The model under review builds one solid part; all positions refer to its coordinate system, in mm. A direction names the side the tool comes from. Round coordinates to 2 decimals unless told otherwise and drop trailing zeros. Write each loop counter-clockwise with the first axis right and the second up, starting at its lowest first coordinate (ties: lowest second). Pieces come first, ordered by that corner, then holes. Notation, with made-up numbers: (73, 59) - (111, 59) arc R18 ccw to (111, 91) - close; hole circle Ø4 at (-32.75, 71.5). An arc over 180 degrees is marked (long way). Use one line per item in the form item = value.
Autodesk Inventor part; units mm, degrees
ref_plane "YZ Plane" through (0, 0, 0) normal (1, 0, 0) x (0, 1, 0)
ref_plane "XZ Plane" through (0, 0, 0) normal (0, 1, 0) x (-1, 0, 0)
ref_plane "XY Plane" through (0, 0, 0) normal (0, 0, 1) x (1, 0, 0)
sketch "Sketch1" plane through (0, 0, 0) normal (0, 1, 0) x (-1, 0, 0)
  line L0 (0, 0) -> (-200, 0)
  line L1 (-200, 0) -> (-200, -150)
  line L2 (-200, -150) -> (0, -150)
  line L3 (0, -150) -> (0, 0)
  line L4 (-109.8726, -150) -> (-90.1274, -150)
  line L5 (-200, -85.1274) -> (-200, -64.8726)
  line L6 (-186.0054, -60.2304) -> (-186.0054, -75)
  line L7 (-200, -64.8726) -> (-187.7125, -59.1428)
  arc A0 (-186.0054, -60.2304) -> (-187.7125, -59.1428) centre (-187.2054, -60.2304) ccw
  line L8 (-186.0054, -75) -> (-186.0054, -89.7696)
  line L9 (-199.8, -85) -> (-186.3697, -85) construction
  arc A1 (-187.7125, -90.8572) -> (-186.0054, -89.7696) centre (-187.2054, -89.7696) ccw
  line L10 (-187.7125, -90.8572) -> (-200, -85.1274)
  line L11 (-89.8726, -150) -> (-110.1274, -150)
  line L12 (-114.7696, -136.0054) -> (-100, -136.0054)
  line L13 (-110.1274, -150) -> (-115.8572, -137.7125)
  arc A2 (-114.7696, -136.0054) -> (-115.8572, -137.7125) centre (-114.7696, -137.2054) ccw
  line L14 (-100, -136.0054) -> (-85.2304, -136.0054)
  line L15 (-90, -149.8) -> (-90, -136.3697) construction
  arc A3 (-84.1428, -137.7125) -> (-85.2304, -136.0054) centre (-85.2304, -137.2054) ccw
  line L16 (-84.1428, -137.7125) -> (-89.8726, -150)
  line L17 (-90.1274, 0) -> (-109.8726, 0)
  line L18 (-85.2304, -13.9946) -> (-100, -13.9946)
  arc A4 (-115.8572, -12.2875) -> (-114.7696, -13.9946) centre (-114.7696, -12.7946) ccw
  arc A5 (-85.2304, -13.9946) -> (-84.1428, -12.2875) centre (-85.2304, -12.7946) ccw
  line L19 (-89.8726, 0) -> (-84.1428, -12.2875)
  line L20 (-110.1274, 0) -> (-89.8726, 0)
  line L21 (-110, -0.2) -> (-110, -13.6303) construction
  line L22 (-115.8572, -12.2875) -> (-110.1274, 0)
  line L23 (-100, -13.9946) -> (-114.7696, -13.9946)
  point P0 (-100, -150)
  point P1 (-100, -150)
  point P2 (-100, -150)
  point P3 (-100, -150)
  point P4 (-200, -75)
  point P5 (-186.2054, -91.3393)
  point P6 (-200, -75)
  point P7 (-200, -75)
  point P8 (-100, -150)
  point P9 (-83.6607, -136.2054)
  point P10 (-100, 0)
  point P11 (-116.3393, -13.7946)
  point P12 (-100, 0)
  point P13 (-100, 0)
  dimension "d0" = 200
  dimension "d1" = 150
  dimension "d2" = 15
  dimension "d13" = 15
  dimension "d14" = 15
extrude "Extrusion1" add sketch "Sketch1" along normal blind 35
extrude "Extrusion2" cut sketch "Sketch1" along normal blind 5.2 contours L7 A0 L6 L8 A1 L10 L1
sketch "Sketch2" plane through (0, 35, 0) normal (0, 1, 0) x (1, 0, 0)
  line L0 (0, 150) -> (0, 0)
  line L1 (0, 75) -> (100, 75)
  circle A0 centre (100, 75) radius 2.6
  dimension "d9" = 100
  dimension "d10" = 5.2
extrude "Extrusion4" cut sketch "Sketch2" against normal blind 5.2
extrude "Extrusion5" cut sketch "Sketch1" along normal blind 4.8 contours L19 A5 L18 L23 A4 L22 L0 | L2 L13 A2 L12 L14 A3 L16
sketch "Sketch3" plane through (0, 0, 0) normal (0, -1, 0) x (1, 0, 0)
  line L0 (200, -150) -> (0, -150)
  line L1 (0, 0) -> (70, 0)
  line L2 (70, 0) -> (70, -150)
  line L3 (70, -150) -> (0, -150)
  line L4 (0, -150) -> (0, 0)
  line L5 (200, 0) -> (200, -64.8726)
  line L6 (200, 0) -> (130, 0)
  line L7 (130, 0) -> (130, -50)
  line L8 (130, -50) -> (200, -50)
  line L9 (200, -50) -> (200, 0)
  line L10 (200, -150) -> (130, -150)
  line L11 (130, -150) -> (130, -100)
  line L12 (130, -100) -> (200, -100)
  line L13 (200, -100) -> (200, -150)
  dimension "d17" = 70
  dimension "d18" = 70
  dimension "d19" = 50
  dimension "d20" = 70
  dimension "d21" = 50
extrude "Extrusion6" cut sketch "Sketch3" against normal blind 40
fillet "Fillet1" radius 10 8 edges at (130, 17.5, -50) (200, 17.5, -50) (200, 17.5, -100) (130, 17.5, 0) (70, 17.5, 0) (70, 17.5, -150) (130, 17.5, -150) (130, 17.5, -100)
properties part number "Area mv"
(1) Add section D-D on x = 178. Write out the cut boundary in (y, z), then the cut area to 3 significant figures.
Geometry results:
outline = (0, -100) - (35, -100) - (35, -50) - (0, -50) - close
area = 1,750 mm2
(2) Add section A-A on x = 100. Write out the cut boundary in (y, z).
Geometry results:
outline = (0, -136.01) - (4.8, -136.01) - (4.8, -150) - (35, -150) - (35, -77.6) - (29.8, -77.6) - (29.8, -72.4) - (35, -72.4) - (35, 0) - (4.8, 0) - (4.8, -13.99) - (0, -13.99) - close
(3) To check wall thickness, follow L1, parallel to Z at x = 100, y = 33.8; L2, parallel to Z at x = 165.5, y = 8.5; L3, parallel to X at y = 10.5, z = -17. State the ranges of each line that lie inside material, in increasing order.
Geometry results:
L1 = -150 to -77.6, -72.4 to 0
L2 = -100 to -50
L3 = 70 to 130
(4) Insertion check: P1, Ø4, axis at x = 102, y = 3, coming from the +Z side; P2, Ø2.5, axis at y = 3.5, z = -68.5, coming from the +X side; P3, Ø17.5, axis at x = 160, y = 22, coming from the +Z side; P4, Ø2.5, axis at x = 95.5, y = 3, coming from the -Z side. Each pin has a flat end and moves straight along its axis. Give the tip position at first contact, or say it passes through.
Geometry results:
P1 = 0
P2 = 186.01
P3 = -50
P4 = -136.01
(5) Machinability: for faces 4 (the flat face through (100, 2, -13.995)), 5 (the cylindrical face through (72.85, 17.74, -3.01)), 6 (the flat face through (165, 17, -50)), which of the approach directions +Z, -Z, +X, -X, +Y, -Y give a long, thin tool a straight path to every point of the face, cutting with its end or side? Answer none if there is none.
Geometry results:
face_4 = -Y
face_5 = +Z, -X, +Y, -Y
face_6 = +Z, +X, +Y, -Y
(6) The part is to be moulded in two halves that separate along X. For faces 1 (the flat face through (165, 17, -100)), 2 (the cylindrical face through (132.85, 17.74, -103.01)), 3 (the cylindrical face through (99.662, 32.436, -77.578)), say which applies: +X half, -X half, draft (parallel to the pull), parting line (faces both ways), or undercut.
Geometry results:
face_1 = draft
face_2 = +X half
face_3 = undercut
(7) Add section C-C on y = 17.5. Write out the cut boundary in (x, z).
Geometry results:
outline = (70, -140) arc R10 ccw to (80, -150) - (120, -150) arc R10 ccw to (130, -140) - (130, -110) arc R10 cw to (140, -100) - (190, -100) arc R10 ccw to (200, -90) - (200, -60) arc R10 ccw to (190, -50) - (140, -50) arc R10 cw to (130, -40) - (130, -10) arc R10 ccw to (120, 0) - (80, 0) arc R10 ccw to (70, -10) - close
(8) Add section B-B on z = -75. Write out the cut boundary in (x, y), then the cut area to 3 significant figures.
Geometry results:
outline = (70, 0) - (186.01, 0) - (186.01, 5.2) - (200, 5.2) - (200, 35) - (102.6, 35) - (102.6, 29.8) - (97.4, 29.8) - (97.4, 35) - (70, 35) - close
area = 4,450 mm2
